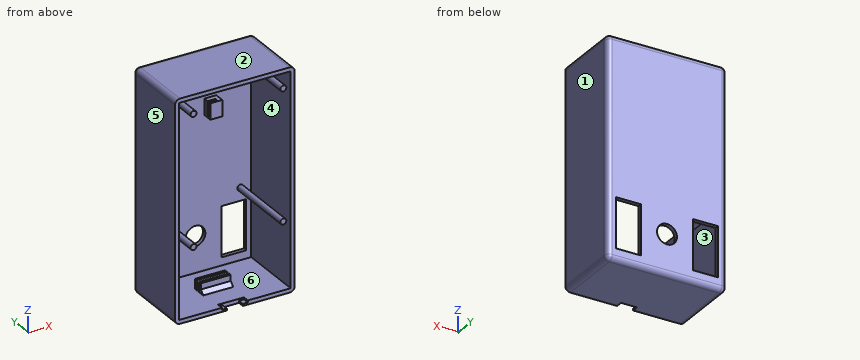
from build123d import *

# Parameters (mm, degrees)
SKETCH1_W           = 60
SKETCH1_H           = 110
BOSS_EXTRUDE1_DEPTH = 35
SKETCH2_W           = 56
SKETCH2_H           = 106
CUT_EXTRUDE1_DEPTH  = 33
SKETCH3_R           = 1.5
BOSS_EXTRUDE2_DEPTH = 36
CUT_EXTRUDE2_DEPTH  = 21
SKETCH6_R           = 5
CUT_EXTRUDE3_DEPTH  = 21
SKETCH7_W           = 8
SKETCH7_H           = 3.25
CUT_EXTRUDE4_DEPTH  = 21
SKETCH8_W           = 13
SKETCH8_H           = 1
CUT_EXTRUDE5_DEPTH  = 3.25
FILLET1_R           = 2.5
SKETCH9_W           = 6
SKETCH9_H           = 8
BOSS_EXTRUDE3_DEPTH = 5
SKETCH10_W          = 18
SKETCH10_H          = 20
CUT_EXTRUDE6_DEPTH  = 1.35
SKETCH11_W          = 4.702418378
SKETCH11_H          = 7.605650594
CUT_EXTRUDE7_DEPTH  = 1.35
SKETCH13_W          = 15
SKETCH13_H          = 1.5
BOSS_EXTRUDE4_DEPTH = 5
CHAMFER1_SIZE       = 2
CUT_EXTRUDE9_START  = -5
SKETCH14_W          = 1
SKETCH14_H          = 3
CUT_EXTRUDE9_DEPTH  = 5


with BuildPart() as part:
    # Sketch1 → Boss-Extrude1 (new body)
    with BuildSketch(Plane(origin=(0, 0, 0), x_dir=(1, 0, 0), z_dir=(0, 1, 0))):
        with Locations((30, 55)):
            Rectangle(SKETCH1_W, SKETCH1_H)
    extrude(amount=BOSS_EXTRUDE1_DEPTH)

    # Sketch2 → Cut-Extrude1 (cut)
    with BuildSketch(Plane.XZ):
        with Locations((30, -55)):
            Rectangle(SKETCH2_W, SKETCH2_H)
    extrude(amount=-CUT_EXTRUDE1_DEPTH, mode=Mode.SUBTRACT)

    # Sketch3 → Boss-Extrude2 (add)
    with BuildSketch(Plane.XZ.offset(-33)):
        with Locations(Location((7.5, -7.5, 0), (0, 0, 270))):
            Circle(SKETCH3_R)
        with Locations(Location((52.5, -7.5, 0), (0, 0, 270))):
            Circle(SKETCH3_R)
        with Locations(Location((7.5, -72.5, 0), (0, 0, 270))):
            Circle(SKETCH3_R)
        with Locations(Location((52.5, -72.5, 0), (0, 0, 270))):
            Circle(SKETCH3_R)
    extrude(amount=BOSS_EXTRUDE2_DEPTH)

    # Sketch4 → Cut-Extrude2 (cut)
    with BuildSketch(Plane(origin=(0, 35, 0), x_dir=(1, 0, 0), z_dir=(0, 1, 0))):
        Polygon((4.5, 104), (17, 104), (17, 85.965044769), (17, 79), (4.5, 79), align=None)
        Polygon((43, 104), (55.5, 104), (55.5, 79), (43, 79), (43, 85.965044769), align=None)
    extrude(amount=-CUT_EXTRUDE2_DEPTH, mode=Mode.SUBTRACT)

    # Sketch6 → Cut-Extrude3 (cut)
    with BuildSketch(Plane(origin=(0, 35, 0), x_dir=(1, 0, 0), z_dir=(0, 1, 0))):
        with Locations(Location((30, 90, 0), (0, 0, 270))):
            Circle(SKETCH6_R)
    extrude(amount=-CUT_EXTRUDE3_DEPTH, mode=Mode.SUBTRACT)

    # Sketch7 → Cut-Extrude4 (cut)
    with BuildSketch(Plane(origin=(0, 0, -110), x_dir=(-1, 0, 0), z_dir=(0, 0, -1))):
        with Locations((-30, 1.625)):
            Rectangle(SKETCH7_W, SKETCH7_H)
    extrude(amount=-CUT_EXTRUDE4_DEPTH, mode=Mode.SUBTRACT)

    # Sketch8 → Cut-Extrude5 (cut)
    with BuildSketch(Plane.XZ):
        with Locations((30, -108.5)):
            Rectangle(SKETCH8_W, SKETCH8_H)
    extrude(amount=-CUT_EXTRUDE5_DEPTH, mode=Mode.SUBTRACT)

    # Fillet1
    fillet1_edges = [part.edges().sort_by_distance(p)[0] for p in [
        (60, 35, -55),
        (30, 35, -110),
        (0, 35, -55),
        (0, 17.5, -110),
        (60, 17.5, -110),
        (60, 17.5, 0),
        (0, 17.5, 0),
        (30, 35, 0),
    ]]
    fillet(fillet1_edges, radius=FILLET1_R)

    # Sketch9 → Boss-Extrude3 (add)
    with BuildSketch(Plane.XZ.offset(-33)):
        Polygon((19.5, -10.111573996), (19.5, -16.111573996), (24.5, -16.111573996), (24.5, -13.111573996), (34.5, -13.111573996), (34.5, -18.111573996), (40.5, -18.111573996), (40.5, -10.111573996), align=None)
        with Locations((37.5, -28.111573996)):
            Rectangle(SKETCH9_W, SKETCH9_H)
    extrude(amount=BOSS_EXTRUDE3_DEPTH)

    # Sketch10 → Cut-Extrude6 (cut)
    with BuildSketch(Plane(origin=(0, 29, 0), x_dir=(-1, 0, 0), z_dir=(0, -1, 0))):
        with Locations((-29.5, 21.111573996)):
            Rectangle(SKETCH10_W, SKETCH10_H)
    extrude(amount=-CUT_EXTRUDE6_DEPTH, mode=Mode.SUBTRACT)

    # Sketch11 → Cut-Extrude7 (cut)
    with BuildSketch(Plane.XZ.offset(-30.35)):
        with Locations((19.397015068, -14.914399293)):
            Rectangle(SKETCH11_W, SKETCH11_H)
    extrude(amount=CUT_EXTRUDE7_DEPTH, mode=Mode.SUBTRACT)

    # Sketch13 → Boss-Extrude4 (add)
    with BuildSketch(Plane.XY.offset(-108)):
        with Locations((29.888929183, 19.75)):
            Rectangle(SKETCH13_W, SKETCH13_H)
        with Locations((29.888929183, 16.5)):
            Rectangle(SKETCH13_W, SKETCH13_H)
    extrude(amount=BOSS_EXTRUDE4_DEPTH)

    # Chamfer1
    chamfer1_edges = [part.edges().sort_by_distance(p)[0] for p in [
        (29.888929183, 15.75, -108),
    ]]
    chamfer(chamfer1_edges, length=CHAMFER1_SIZE)

    # Sketch14 → Cut-Extrude9 (cut)
    with BuildSketch(Plane.XZ.offset(-28).offset(CUT_EXTRUDE9_START)):
        with Locations((24, -14.611573996)):
            Rectangle(SKETCH14_W, SKETCH14_H)
    extrude(amount=CUT_EXTRUDE9_DEPTH, mode=Mode.SUBTRACT)


solid = part.part
For this review, take the finished solid that the model builds, in its own axes (mm). Face numbers are marked on the shaded views. A direction names the side the tool comes from. Give positions to 0.01 mm unless a question says otherwise; leave off trailing zeros. Loops run counter-clockwise (first coordinate to the right, second up) from the corner with the lowest first, then second, coordinate; pieces in that order, holes last. Notation, with made-up numbers: M -35,-34 L -14,-34 A15 cw -14,-29 Z; hole C 33.25,65 d10. An arc over 180 degrees is marked long. Put each result on its own line as item: value. Start each with the question number.
(1) Add section B-B, the plane x = 7.5. Write out the cut boundary in (y, z).
(2) For pin 1 (2 mm diameter, centred on x = 10.5, y = 34.5, fed in from -Z); pin 2 (8 mm diameter, centred on x = 6.5, z = -19.5, fed in from -Y); pin 3 (2 mm diameter, centred on y = 34, z = -87, fed in from +X), all flat-tipped, find the tip position at first contact; note any pin that passes through.
(3) Add section C-C, the plane z = -100. Write out the cut boundary in (x, y).
(4) Add section D-D, the plane z = -72.5. Write out the cut boundary in (x, y).
(5) The part is to be moulded in two halves that separate along X. For the marked faces 1, 2 and 3, say which applies: +X half, -X half, draft (parallel to the pull), parting line (faces both ways), or undercut.
(6) Add section A-A, the plane y = 26.5. Write out the cut boundary in (x, z).
(7) Machinability: for the marked faces 4, 5 and 6, which of the approach directions +Z, -Z, +X, -X, +Y, -Y give a long, thin tool a straight path to every point of the face, cutting with its end or side? Answer none if there is none.
(8) Wall thickness on L1, parallel to Z at x = 28.5, y = 27.5; L2, parallel to Z at x = 31.5, y = 32.5; L3, parallel to X at y = 18, z = -85.5: over which ranges is each line inside the solid? List them lowest first.
Result:
1. outline: M -3,-74 L 33,-74 L 33,-79 L 35,-79 L 35,-2.5 A2.5 ccw 32.5,0 L 0,0 L 0,-2 L 33,-2 L 33,-6 L -3,-6 L -3,-9 L 33,-9 L 33,-71 L -3,-71 Z; M 0,-110 L 32.5,-110 A2.5 ccw 35,-107.5 L 35,-104 L 33,-104 L 33,-108 L 0,-108 Z
2. pin 1: stops at z = -109.79
2. pin 2: stops at y = 33
2. pin 3: stops at x = 59.95
3. outline: M 0,0 L 2,0 L 2,33 L 4.5,33 L 4.5,35 L 2.5,35 A2.5 ccw 0,32.5 Z; M 17,33 L 43,33 L 43,35 L 17,35 Z; M 55.5,33 L 58,33 L 58,0 L 60,0 L 60,32.5 A2.5 ccw 57.5,35 L 55.5,35 Z
4. outline: M 0,0 L 2,0 L 2,33 L 6,33 L 6,-3 L 9,-3 L 9,33 L 51,33 L 51,-3 L 54,-3 L 54,33 L 58,33 L 58,0 L 60,0 L 60,32.5 A2.5 ccw 57.5,35 L 2.5,35 A2.5 ccw 0,32.5 Z
5. face 1: +X half
5. face 2: draft
5. face 3: undercut
6. outline: M 0,-107.5 A2.5 ccw 2.5,-110 L 57.5,-110 A2.5 ccw 60,-107.5 L 60,-2.5 A2.5 ccw 57.5,0 L 2.5,0 A2.5 ccw 0,-2.5 Z; C 7.5,-72.5 d3; C 7.5,-7.5 d3; C 52.5,-72.5 d3; C 52.5,-7.5 d3; hole M 2,-108 L 58,-108 L 58,-2 L 2,-2 Z
7. face 4: -Y
7. face 5: +Z, -Z, -X, +Y, -Y
7. face 6: none
8. L1: z = -110 to -108, -2 to 0
8. L2: z = -110 to -108, -13.11 to -10.11, -2 to 0
8. L3: x = 0 to 2, 58 to 60
